Work out the finished part from the listing and answer in its coordinate system (mm). A direction names the side the tool comes from. Coordinates: 2 decimals unless noted, no trailing zeros. Loops run counter-clockwise (first coordinate to the right, second up) from the corner with the lowest first, then second, coordinate; pieces in that order, holes last. Notation, with made-up numbers: (72.25, -27) -> (112.25, -27) arc R25 cw to (112.25, 9) -> close; hole circle Ø3 at (56, -12.5). An arc over 180 degrees is marked (long way). Answer as CSV lines item,"result".
```python
from build123d import *

# Parameters (mm, degrees)
F0_W     = 20
F0_H     = 29
F1_DEPTH = 11
F2_W     = 16
F2_H     = 30
F3_DEPTH = 3
F5_DEPTH = 6.5
F7_DEPTH = 9
F8_R     = 4
F9_R     = 7
F10_R    = 0.5


with BuildPart() as f1:
    # F0 (on Front) → F1 (new body)
    with BuildSketch(Plane.XZ):
        Rectangle(F0_W, F0_H)
    extrude(amount=F1_DEPTH)

    # F2 (on face) → F3 (cut)
    with BuildSketch(Plane.XZ):
        with Locations((0, 2.5)):
            Rectangle(F2_W, F2_H)
    extrude(amount=F3_DEPTH, mode=Mode.SUBTRACT)

    # F4 (on face) → F5 (cut)
    with BuildSketch(Plane(origin=(0, -3, 0), x_dir=(-1, 0, 0), z_dir=(0, 1, 0))):
        with BuildLine():
            Line((0, -8.15), (0.659236, -8.715135))
            ThreePointArc((0.659236, -8.715135), (5.412659, -5.625), (5.712083, 0.036653))
            Line((5.712083, 0.036653), (4.893044, 0.325))
            Line((4.893044, 0.325), (5.052847, 1.178482))
            ThreePointArc((5.052847, 1.178482), (0, 3.75), (-5.052847, 1.178482))
            Line((-5.052847, 1.178482), (-4.893044, 0.325))
            Line((-4.893044, 0.325), (-5.712083, 0.036653))
            ThreePointArc((-5.712083, 0.036653), (-5.412659, -5.625), (-0.659236, -8.715135))
            Line((-0.659236, -8.715135), (0, -8.15))
        make_face()
    extrude(amount=-F5_DEPTH, mode=Mode.SUBTRACT)

    # F6 (on face) → F7 (cut)
    with BuildSketch(Plane.XY.offset(14.5)):
        with BuildLine():
            ThreePointArc((-3.354102, -3), (-1.605699, -10.203776), (4.5, -6))
            ThreePointArc((4.5, -6), (4.203776, -4.394301), (3.354102, -3))
            Line((3.354102, -3), (-3.354102, -3))
        make_face()
    extrude(amount=-F7_DEPTH, mode=Mode.SUBTRACT)

    # F8
    f8_edges = [f1.edges().sort_by_distance(p)[0] for p in [
        (8, -1.5, -12.5),
        (-8, -1.5, -12.5),
    ]]
    fillet(f8_edges, radius=F8_R)

    # F9
    f9_edges = [f1.edges().sort_by_distance(p)[0] for p in [
        (-10, -5.5, -14.5),
        (10, -5.5, -14.5),
        (0, -11, -14.5),
        (10, -11, 0),
        (-10, -11, 0),
    ]]
    fillet(f9_edges, radius=F9_R)

    # F10
    f10_edges = [f1.edges().sort_by_distance(p)[0] for p in [
        (8, -3, 3),
        (10, 0, 3.5),
    ]]
    fillet(f10_edges, radius=F10_R)


solid = f1.part
```
(1) A cutting plane is placed at D-D, the plane z = 2.25. Write down the section's boundary in (x, y), and give its area (3 significant figures).
Computed values:
outline,"(-10, -4) arc R7 ccw to (-3, -11) -> (3, -11) arc R7 ccw to (10, -4) -> (10, -0.5) arc R0.5 ccw to (9.5, 0) -> (8, 0) -> (8, -2.5) arc R0.5 cw to (7.5, -3) -> (4.06, -3) -> (4.06, -9.5) -> (-4.06, -9.5) -> (-4.06, -3) -> (-7.5, -3) arc R0.5 cw to (-8, -2.5) -> (-8, 0) -> (-9.5, 0) arc R0.5 ccw to (-10, -0.5) -> close"
area,"98.2 mm2"
(2) A cutting plane is placed at A-A, the plane y = -8. Write down the section's boundary in (x, z) (3 decimals), and give its area (3 significant figures).
Computed values:
outline,"(-8.745, -7.5) arc R5.745 ccw to (-3, -13.245) -> (3, -13.245) arc R5.745 ccw to (8.745, -7.5) -> (8.745, 14.5) -> (4.031, 14.5) -> (4.031, 5.5) -> (-4.031, 5.5) -> (-4.031, 14.5) -> (-8.745, 14.5) -> close; hole (-5.712, 0.037) arc R6.25 ccw to (-0.659, -8.715) -> (0, -8.15) -> (0.659, -8.715) arc R6.25 ccw to (5.712, 0.037) -> (4.893, 0.325) -> (5.053, 1.178) arc R6.25 ccw to (-5.053, 1.178) -> (-4.893, 0.325) -> close"
area,"277 mm2"
(3) A cutting plane is placed at C-C, the plane z = 10. Write down the section's boundary in (x, y), and give its area (3 significant figures).
Computed values:
outline,"(-10, -4) arc R7 ccw to (-3, -11) -> (3, -11) arc R7 ccw to (10, -4) -> (10, -0.5) arc R0.5 ccw to (9.5, 0) -> (8, 0) -> (8, -2.5) arc R0.5 cw to (7.5, -3) -> (3.35, -3) arc R4.5 cw to (4.5, -6) arc R4.5 cw (long way) to (-3.35, -3) -> (-7.5, -3) arc R0.5 cw to (-8, -2.5) -> (-8, 0) -> (-9.5, 0) arc R0.5 ccw to (-10, -0.5) -> close"
area,"94.3 mm2"
(4) Consider line 1 along X through (y, z) = (-1.75, -3.75); line 2 along X through (y, z) = (-2.5, -10.75); line 3 along Y through (x, z) = (-4, 5.75). Determine where each line is inside the solid, lowest interval first.
Computed values:
line 1,"-10 to -8, 8 to 10"
line 2,"-9.2 to -7.31, 7.31 to 9.2"
line 3,"-10.93 to -8.06, -3.94 to -3"
(5) For a pull along X with two mould halves and no side action, classify faces 1 (the face through (7.9, -2.3, -12.5)), 2 (the face through (-8, -2.3, -12.4)), 3 (the face through (8, -1, 3)), 4 (the face through (-8.5, 0, -1.8)) as pulls with the +X half, pulls with the -X half, needs draft (parallel to the pull), parting line crosses it, or undercut.
Computed values:
face 1,"pulls with the +X half"
face 2,"pulls with the -X half"
face 3,"undercut"
face 4,"needs draft"
(6) A cutting plane is placed at B-B, the plane z = -3.25. Write down the section's boundary in (x, y), and give its area (3 significant figures).
Computed values:
outline,"(-10, -4) arc R7 ccw to (-3, -11) -> (3, -11) arc R7 ccw to (10, -4) -> (10, -0.5) arc R0.5 ccw to (9.5, 0) -> (8, 0) -> (8, -2.5) arc R0.5 cw to (7.5, -3) -> (6.2, -3) -> (6.2, -9.5) -> (-6.2, -9.5) -> (-6.2, -3) -> (-7.5, -3) arc R0.5 cw to (-8, -2.5) -> (-8, 0) -> (-9.5, 0) arc R0.5 ccw to (-10, -0.5) -> close"
area,"70.3 mm2"
(7) Flat-ended cylindrical pins translate along their axes: pin 1 Ø2 at (y, z) = (-7, 9.5) entering from +X; pin 2 Ø6 at (x, z) = (-1, 0) entering from +Y; pin 3 Ø5 at (x, y) = (-3.5, -8.5) entering from -Z. Find the tip coordinate at first contact, or state that the pin passes through.
Computed values:
pin 1,"x = 9.71"
pin 2,"y = -9.5"
pin 3,"z = -14.2"
(8) Which of the six approach directions +Z, -Z, +X, -X, +Y, -Y give full straight-line access (tool end or side, diameter ignored) to faces 5 (the face through (0, -7, 5.5)), 6 (the face through (0, -9.5, -2)), 7 (the face through (-5, -7, 14.5)), 8 (the face through (10, -2, 3)), 9 (the face through (0, -3, 4))?
Computed values:
face 5,"+Z"
face 6,"+Y"
face 7,"+Z, +X, -X, +Y, -Y"
face 8,"+Z, -Z, +X, +Y, -Y"
face 9,"+Z, +Y"
